```python
from build123d import *

# Parameters (mm, degrees)
SKETCH2_R          = 5.05
CUT_EXTRUDE1_DEPTH = 71.887234394
CHAMFER1_SIZE      = 1


with BuildPart() as part:
    # Sketch1 → Revolve1 (revolve)
    with BuildSketch(Plane.XY, mode=Mode.PRIVATE) as revolve1_sk:
        Polygon((0, 0), (20, 0), (20, -45), (12, -45), (12, -65), (0, -65), align=None)
    revolve(revolve1_sk.sketch.rotate(Axis((0, -70, 0), (0, 1, 0)), 90), axis=Axis((0, -70, 0), (0, 1, 0)))

    # Sketch2 → Cut-Extrude1 (cut, through all)
    with BuildSketch(Plane(origin=(0, 0, 0), x_dir=(1, 0, 0), z_dir=(0, 1, 0))):
        with Locations(Location((0, 0, 0), (0, 0, 180))):
            Circle(SKETCH2_R)
    extrude(amount=-CUT_EXTRUDE1_DEPTH, mode=Mode.SUBTRACT)

    # Chamfer1
    chamfer1_edges = [part.edges().sort_by_distance(p)[0] for p in [
        (5.05, -65, 0),
        (5.05, 0, 0),
        (0, -65, 12),
        (0, -45, 20),
        (0, 0, 20),
    ]]
    chamfer(chamfer1_edges, length=CHAMFER1_SIZE)


solid = part.part
```
For this review, take the finished solid that the model builds, in its own axes (mm). A direction names the side the tool comes from. Round coordinates to 2 decimals unless told otherwise and drop trailing zeros. Write each loop counter-clockwise with the first axis right and the second up, starting at its lowest first coordinate (ties: lowest second). Pieces come first, ordered by that corner, then holes. Notation, with made-up numbers: (60.5, 46) -> (110.5, 46) arc R18 cw to (110.5, 71) -> close; hole circle Ø9 at (40.25, 36). An arc over 180 degrees is marked (long way). Use one line per item in the form item = value.
Q1. To check wall thickness, follow probe 1 along Y at (x, z) = (2, -15); probe 2 along X at (y, z) = (-24.5, -2); probe 3 along Z at (x, y) = (-1, -36.5). State the ranges of each line that lie inside material, in increasing order. Write a range as from..to.
Resolved:
probe_1 = -45..0
probe_2 = -19.9..-4.64, 4.64..19.9
probe_3 = -19.97..-4.95, 4.95..19.97
Q2. The part is to be moulded in two halves that separate along X. For faces 3 (the cylindrical face through (4.01, -32.06, -3.07)), 4 (the flat face through (-4.5, 0, -4.5)), 5 (the cylindrical face through (-0.88, -22.8, 19.98)), say which applies: released by +X, released by -X, zero draft, split by the parting line, or undercut.
Resolved:
face_3 = undercut
face_4 = zero draft
face_5 = split by the parting line
Q3. Consider section D-D (y = -21). State the section outline as (x, z) points.
Resolved:
outline = circle Ø40 at (0, 0); hole circle Ø10.1 at (0, 0)
Q4. Consider section A-A (x = 0). State the section outline as (y, z) points, then the cut area to 3 significant figures.
Resolved:
outline = (-65, -11) -> (-64, -12) -> (-45, -12) -> (-45, -19) -> (-44, -20) -> (-1, -20) -> (0, -19) -> (0, -6.05) -> (-1, -5.05) -> (-64, -5.05) -> (-65, -6.05) -> close; (-65, 6.05) -> (-64, 5.05) -> (-1, 5.05) -> (0, 6.05) -> (0, 19) -> (-1, 20) -> (-44, 20) -> (-45, 19) -> (-45, 12) -> (-64, 12) -> (-65, 11) -> close
area = 1,620 mm²
Q5. Consider section C-C (y = -54.5). State the section outline as (x, z) points.
Resolved:
outline = circle Ø24 at (0, 0); hole circle Ø10.1 at (0, 0)
Q6. Consider section B-B (z = 0). State the section outline as (x, y) points, then the cut area to 3 significant figures.
Resolved:
outline = (-20, -44) -> (-19, -45) -> (-12, -45) -> (-12, -64) -> (-11, -65) -> (-6.05, -65) -> (-5.05, -64) -> (-5.05, -1) -> (-6.05, 0) -> (-19, 0) -> (-20, -1) -> close; (5.05, -64) -> (6.05, -65) -> (11, -65) -> (12, -64) -> (12, -45) -> (19, -45) -> (20, -44) -> (20, -1) -> (19, 0) -> (6.05, 0) -> (5.05, -1) -> close
area = 1,620 mm²
Q7. Clearance check with flat-ended pins moving along their axes: pin 1 Ø10 at (x, y) = (-16, -25.5) entering from +Z; pin 2 Ø8 at (x, z) = (0, 0) entering from +Y; pin 3 Ø1.5 at (y, z) = (-30, -5.5) entering from +X; pin 4 Ø12 at (x, y) = (10.5, -42) entering from +Z. State where each tip first meets the part, or that it passes through.
Resolved:
pin_1 = 16.7
pin_2 = through
pin_3 = 19.43
pin_4 = 19.49
Q8. Machinability: for faces 1 (the flat face through (5, -65, -5)), 2 (the cylindrical face through (-3.604, -54.633, -11.446)), which of the approach directions +Z, -Z, +X, -X, +Y, -Y give a long, thin tool a straight path to every point of the face, cutting with its end or side? Answer none if there is none.
Resolved:
face_1 = +Z, -Z, +X, -X, -Y
face_2 = -Y
